```python
from build123d import *

# Parameters (mm, degrees)
SKETCH2_W             = 241
SKETCH2_H             = 50
BOSS_EXTRUDE1_DEPTH   = 16
SKETCH3_R             = 10.5
CUT_EXTRUDE1_DEPTH    = 8
SKETCH6_R             = 4.5
CUT_EXTRUDE2_DEPTH    = 124.325788057
M5_TAPPED_HOLE4_D     = 4.2
M5_TAPPED_HOLE4_DEPTH = 22.4
M5_TAPPED_HOLE4_TIP   = 1.2618073


with BuildPart() as part:
    # Sketch2 → Boss-Extrude1 (new body)
    with BuildSketch(Plane(origin=(0, 0, 0), x_dir=(1, 0, 0), z_dir=(0, 1, 0))):
        Rectangle(SKETCH2_W, SKETCH2_H)
    extrude(amount=BOSS_EXTRUDE1_DEPTH)

    # Sketch3 → Cut-Extrude1 (cut)
    with BuildSketch(Plane(origin=(0, 16, 0), x_dir=(1, 0, 0), z_dir=(0, 1, 0))):
        with Locations(Location((-90.5, 0, 0), (0, 0, 270))):
            Circle(SKETCH3_R)
    extrude(amount=-CUT_EXTRUDE1_DEPTH, mode=Mode.SUBTRACT)

    # Sketch6 → Cut-Extrude2 (cut, through all)
    with BuildSketch(Plane(origin=(0, 8, 0), x_dir=(1, 0, 0), z_dir=(0, 1, 0))):
        with Locations(Location((-90.5, 0, 0), (0, 0, 270))):
            Circle(SKETCH6_R)
    extrude(amount=-CUT_EXTRUDE2_DEPTH, mode=Mode.SUBTRACT)

    # M5 Tapped Hole4
    with Locations(Plane(origin=(120.5, 0, 0), x_dir=(0, 0, -1), z_dir=(1, 0, 0))):
        with Locations((-12.5, 8), (12.5, 8)):
            Hole(M5_TAPPED_HOLE4_D / 2, depth=M5_TAPPED_HOLE4_DEPTH)
            with Locations((0, 0, -(M5_TAPPED_HOLE4_DEPTH + M5_TAPPED_HOLE4_TIP / 2))):  # 118° drill point
                Cone(0, M5_TAPPED_HOLE4_D / 2, M5_TAPPED_HOLE4_TIP, mode=Mode.SUBTRACT)


solid = part.part
```
Design review of the part built by this model. Coordinates are the model's own, in mm. A direction names the side the tool comes from. Round coordinates to 2 decimals unless told otherwise and drop trailing zeros. Order: outer loops, then holes, each group sorted by start corner. A loop starts at its lowest first (then second) coordinate and runs counter-clockwise, first axis right, second up. Notation, with made-up numbers: (27, 21) - (41, 21) arc R32 cw to (41, 51) - close; hole circle Ø3 at (66.5, 11.25). An arc over 180 degrees is marked (long way). Return JSON: item names as keys, results as strings.
Q1. For pin 1 Ø12.5 at (x, z) = (-90.5, 0) entering from +Y; pin 2 Ø4 at (y, z) = (8, 12.5) entering from +X, all flat-tipped, find the tip position at first contact; note any pin that passes through.
Computed values:
{"pin 1": "stops at y = 8", "pin 2": "stops at x = 98.04"}
Q2. Machinability: for faces 1 (the cylindrical face through (109.143, 10.082, -12.773)), 2 (the flat face through (-90, 8, 5)), 3 (the flat face through (-2, 16, 0)), which of the approach directions +Z, -Z, +X, -X, +Y, -Y give a long, thin tool a straight path to every point of the face, cutting with its end or side? Answer none if there is none.
Computed values:
{"face 1": "+X", "face 2": "+Y", "face 3": "+Z, -Z, +X, -X, +Y"}
Q3. Consider section B-B on x = -88. Write out the cut boundary in (y, z).
Computed values:
{"outline": "(0, -25) - (16, -25) - (16, -10.2) - (8, -10.2) - (8, -3.74) - (0, -3.74) - close; (0, 3.74) - (8, 3.74) - (8, 10.2) - (16, 10.2) - (16, 25) - (0, 25) - close"}
Q4. Wall thickness on L1, parallel to Z at x = 108.5, y = 8; L2, parallel to X at y = 13.75, z = 0; L3, parallel to X at y = 4.75, z = 0: over which ranges is each line inside the solid? List them lowest first. Write a range as [from, to].
Computed values:
{"L1": "z = [-25, -14.6], [-10.4, 10.4], [14.6, 25]", "L2": "x = [-120.5, -101], [-80, 120.5]", "L3": "x = [-120.5, -95], [-86, 120.5]"}
Q5. The part is to be moulded in two halves that separate along Z. For faces 4 (the flat face through (-2, 0, 0)), 5 (the conical face through (97.057, 8.362, -12.453)), 6 (the flat face through (-2, 8, -25)), say which applies: pulls with the +Z half, pulls with the -Z half, needs draft (parallel to the pull), parting line crosses it, or undercut.
Computed values:
{"face 4": "needs draft", "face 5": "undercut", "face 6": "pulls with the -Z half"}
Q6. Consider section A-A on z = -2. Write out the cut boundary in (x, y).
Computed values:
{"outline": "(-120.5, 0) - (-94.53, 0) - (-94.53, 8) - (-100.81, 8) - (-100.81, 16) - (-120.5, 16) - close; (-86.47, 0) - (120.5, 0) - (120.5, 16) - (-80.19, 16) - (-80.19, 8) - (-86.47, 8) - close"}
